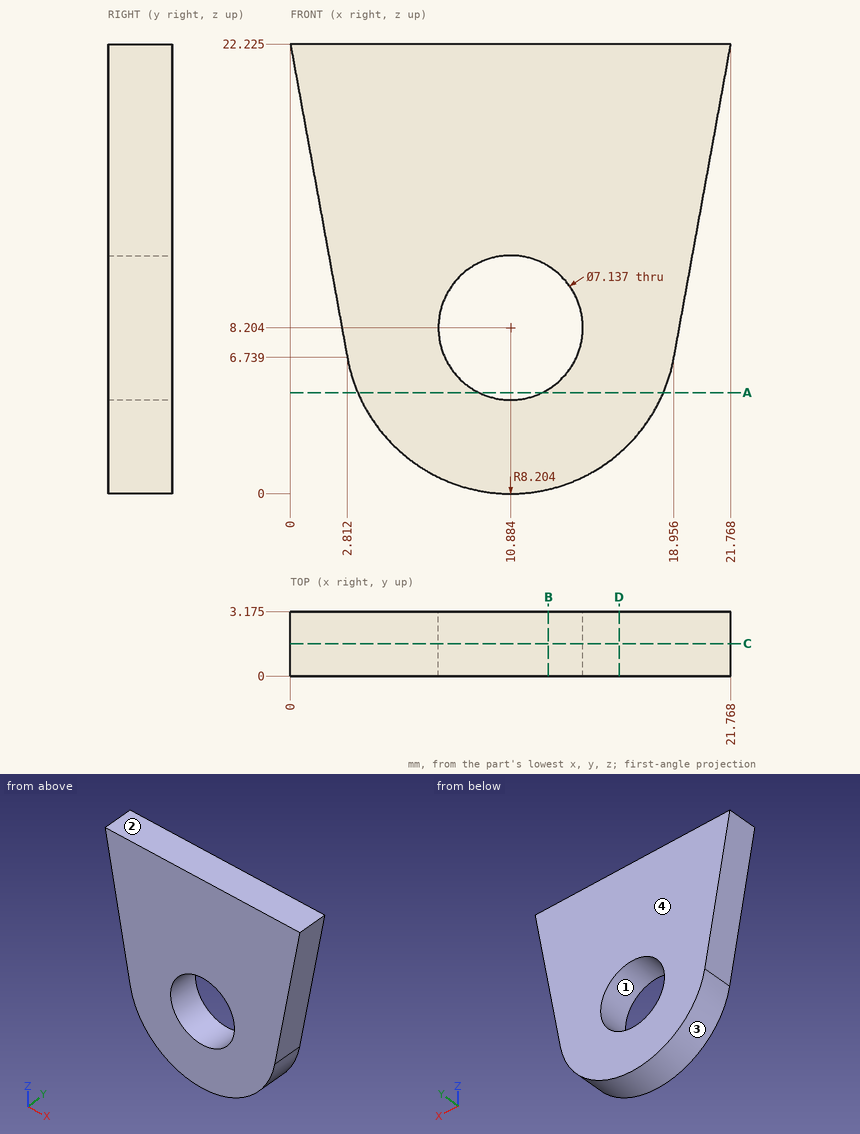
Design review of the part shown in the three views and the two pictorial views. Dimensions are in mm from the part's minimum x, y and z. Give positions to 0.01 mm unless a question says otherwise; leave off trailing zeros. Write each loop counter-clockwise with the first axis right and the second up, starting at its lowest first coordinate (ties: lowest second). Pieces come first, ordered by that corner, then holes. Notation, with made-up numbers: M -4.5,5 L 41.5,5 A20 cw 41.5,44 Z; hole C -27,54.5 d5. An arc over 180 degrees is marked long. Answer in a Markdown table with one row per item.
Item 1: Draft analysis for pull direction Z (two halves, no side actions). For the marked faces 1, 2, 3 and 4, state which applies: +Z half, -Z half, draft (parallel to the pull), parting line (faces both ways), or undercut.
Check sheet entries:
| item | result |
|---|---|
| face 1 | undercut |
| face 2 | +Z half |
| face 3 | -Z half |
| face 4 | draft |
Item 2: For line 1 along Z through (x, y) = (9, 1.4) (1 decimal); line 2 along X through (y, z) = (1.1, 8.5) (1 decimal); line 3 along Z through (x, y) = (7.75, 1) (1 decimal), list the stretches that pass through material, from the lowest coordinate up.
Check sheet entries:
| item | result |
|---|---|
| line 1 | 0.2 to 5.2, 11.2 to 22.2 |
| line 2 | 2.5 to 7.3, 14.4 to 19.3 |
| line 3 | 0.6 to 6.5, 9.9 to 22.2 |
Item 3: Add section A-A on z = 5. Give the boundary of the cut face in (x, y) (1 decimal), plus the area to 3 significant figures.
Check sheet entries:
| item | result |
|---|---|
| outline | M 3.3,0 L 9.3,0 L 9.3,3.2 L 3.3,3.2 Z; M 12.5,0 L 18.4,0 L 18.4,3.2 L 12.5,3.2 Z |
| area | 38.0 mm2 |
Item 4: Add section B-B on x = 12.75. Give the boundary of the cut face in (y, z) (1 decimal).
Check sheet entries:
| item | result |
|---|---|
| outline | M 0,0.2 L 3.2,0.2 L 3.2,5.2 L 0,5.2 Z; M 0,11.2 L 3.2,11.2 L 3.2,22.2 L 0,22.2 Z |
Item 5: For P1, Ø8, axis at x = 5.5, z = 5.5, coming from the -Y side; P2, Ø6.5, axis at x = 10.88, z = 8.2, coming from the -Y side; P3, Ø1, axis at y = 0.5, z = 18, coming from the +X side, all flat-tipped, find the tip position at first contact; note any pin that passes through.
Check sheet entries:
| item | result |
|---|---|
| P1 | y = 0 |
| P2 | through |
| P3 | x = 21.09 |
Item 6: Add section C-C on y = 1.6. Give the boundary of the cut face in (x, z) (1 decimal), plus the area to 3 significant figures.
Check sheet entries:
| item | result |
|---|---|
| outline | M 0,22.2 L 2.8,6.7 A8.2 ccw 19,6.7 L 21.8,22.2 Z; hole C 10.9,8.2 d7.1 |
| area | 335 mm2 |
Item 7: Add section D-D on x = 16.25. Give the boundary of the cut face in (y, z) (1 decimal).
Check sheet entries:
| item | result |
|---|---|
| outline | M 0,2 L 3.2,2 L 3.2,22.2 L 0,22.2 Z |
